Input: part model. Units: mm. Frame: model coordinates. Coordinates: 2 decimals unless noted, no trailing zeros. Order: outer loops, then holes, each group sorted by start corner. A loop starts at its lowest first (then second) coordinate and runs counter-clockwise, first axis right, second up. Notation, with made-up numbers: (71.25, 12) - (95.25, 12) arc R24 ccw to (95.25, 46) - close; hole circle Ø5 at (2.5, 55). An arc over 180 degrees is marked (long way). Answer as CSV lines item,"result". Start each with the question number.
Item 1: Draft query along X for faces 1 (the flat face through (26, 2, 6)), 2 (the cylindrical face through (47.79, -88.63, 2.96)), 3 (the cylindrical face through (-124.88, -5.5, 2.96)). Return one class per face: +X half, -X half, draft (parallel to the pull), parting line (faces both ways), or undercut.
Item 2: First-contact query: pin 1 (3.5 mm diameter, centred on x = -50, y = -86.6, fed in from -Z); pin 2 (1.5 mm diameter, centred on y = -67.5, z = 1, fed in from +X); pin 3 (1 mm diameter, centred on y = -99.5, z = 1.5, fed in from -X); pin 4 (1 mm diameter, centred on x = -27, z = 2, fed in from +Y). Flat tips, straight axial feed; report the tip coordinate or a pass-through.
Item 3: Section B-B (x = -76.95). Output: boundary loops of the cut face in (y, z).
Item 4: Material intervals for line 1 along Y through (x, z) = (-50.5, 0.75); line 2 along X through (y, z) = (41, 4.55); line 3 along Y through (x, z) = (-76.95, 1.75), sorted ascending.
Item 5: Section D-D (x = -50). Output: boundary loops of the cut face in (y, z).
Item 6: Section A-A (y = 0). Output: boundary loops of the cut face in (x, z), and give its area (3 significant figures).
Item 7: Section C-C (z = 1.4). State how many separate pieces and enclosed holes the cut face has, and give its area (3 significant figures).
Autodesk Fusion 360 part; units mm, degrees
sketch "Sketch1" plane through (0, 0, 0) normal (0, 0, 1) x (1, 0, 0)
  circle A0 centre (0, 0) radius 125
  line L0 (0, 0) -> (125, 0)
  line L1 (0, 0) -> (-62.5, -108.2532)
  line L2 (0, 0) -> (-62.5, 108.2532)
  line L3 (0, 0) -> (125, 0) construction
  line L4 (0, 0) -> (-25, 43.3013)
  line L5 (-25, 43.3013) -> (-50, 86.6025)
  line L6 (0, 0) -> (50, 0)
  line L7 (50, 0) -> (100, 0)
  line L8 (0, 0) -> (-25, -43.3013)
  line L9 (-25, -43.3013) -> (-50, -86.6025)
  circle A1 centre (-50, 86.6025) radius 3
  circle A2 centre (-25, 43.3013) radius 3
  circle A3 centre (50, 0) radius 3
  circle A4 centre (100, 0) radius 3
  circle A5 centre (-25, -43.3013) radius 3
  circle A6 centre (-50, -86.6025) radius 3
  line L10 (0, 0) -> (62.5, 108.2532)
  line L11 (0, 0) -> (125, 0) construction
  line L12 (0, 0) -> (62.5, -108.2532)
  line L13 (0, 0) -> (125, 0) construction
  line L14 (0, 0) -> (-125, 0)
  line L15 (0, 0) -> (-100, 0)
  circle A7 centre (-100, 0) radius 3
  line L16 (0, 0) -> (50, -86.6025)
  circle A8 centre (50, -86.6025) radius 3
  line L17 (0, 0) -> (50, 86.6025)
  circle A9 centre (50, 86.6025) radius 3
  circle A10 centre (0, 0) radius 3
  dimension "d1" = 250
  dimension "d2" = 60
  dimension "d3" = 120
  dimension "d4" = 50
  dimension "d5" = 50
  dimension "d6" = 50
  dimension "d7" = 50
  dimension "d8" = 50
  dimension "d9" = 50
  dimension "d10" = 6
  dimension "d11" = 6
  dimension "d12" = 6
  dimension "d13" = 6
  dimension "d14" = 6
  dimension "d15" = 6
  dimension "d16" = 60
  dimension "d17" = 60
  dimension "d18" = 100
  dimension "d19" = 6
  dimension "d20" = 100
  dimension "d21" = 6
  dimension "d22" = 100
  dimension "d23" = 6
  dimension "d24" = 6
extrude "Extrude1" add sketch "Sketch1" along normal blind 6 contours A0 L0 L6 L7 A3 A4 L10 L17 A9 A10 | A0 L0 L6 L7 A3 A4 L12 L16 A8 A10 | A0 L2 L4 L5 A1 A2 L10 L17 A9 A10 | A0 L1 L8 L9 A5 A6 L12 L16 A8 A10 | A0 L2 L4 L5 A1 A2 L14 L15 A7 A10 | A0 L1 L8 L9 A5 A6 L14 L15 A7 A10
sketch "Sketch2" plane through (0, 0, 6) normal (0, 0, 1) x (-1, 0, 0)
  circle A0 centre (0, 0) radius 3
  circle A1 centre (-50, -86.6025) radius 3
  circle A2 centre (25, -43.3013) radius 3
  circle A3 centre (100, 0) radius 3
  circle A4 centre (25, 43.3013) radius 3
  circle A5 centre (50, -86.6025) radius 3
  circle A6 centre (-100, 0) radius 3
  circle A7 centre (-50, 86.6025) radius 3
  circle A8 centre (-50, 0) radius 3
  circle A9 centre (50, 86.6025) radius 3
  circle A10 centre (0, 0) radius 125
  line L0 (125, 0) -> (115, 0)
  circle A11 centre (115, 0) radius 3
  circle A12 centre (105.0577, 46.7747) radius 3
  circle A13 centre (76.95, 85.4617) radius 3
  circle A14 centre (35.537, 109.3715) radius 3
  circle A15 centre (-12.0208, 114.37) radius 3
  circle A16 centre (-57.5, 99.5929) radius 3
  circle A17 centre (-93.037, 67.5953) radius 3
  circle A18 centre (-112.487, 23.9098) radius 3
  circle A19 centre (-112.487, -23.9098) radius 3
  circle A20 centre (-93.037, -67.5953) radius 3
  circle A21 centre (-57.5, -99.5929) radius 3
  circle A22 centre (-12.0208, -114.37) radius 3
  circle A23 centre (35.537, -109.3715) radius 3
  circle A24 centre (76.95, -85.4617) radius 3
  circle A25 centre (105.0577, -46.7747) radius 3
  dimension "d27" = 10
  dimension "d28" = 6
  dimension "d30" = 360
extrude "Extrude2" cut sketch "Sketch2" against normal blind 6 contours A11 | A12 | A13 | A14 | A15 | A16 | A17 | A18 | A19 | A20 | A21 | A22 | A23 | A24 | A25
sketch "Sketch3" plane through (0, 0, 6) normal (0, 0, 1) x (-1, 0, 0)
  circle A0 centre (35.537, 109.3715) radius 3
  circle A1 centre (-112.487, 23.9098) radius 3
  circle A2 centre (-12.0208, -114.37) radius 3
  circle A3 centre (115, 0) radius 3
  circle A4 centre (35.537, -109.3715) radius 3
  circle A5 centre (-112.487, -23.9098) radius 3
  circle A6 centre (-12.0208, 114.37) radius 3
  circle A7 centre (76.95, 85.4617) radius 3
  circle A8 centre (-93.037, 67.5953) radius 3
  circle A9 centre (-57.5, -99.5929) radius 3
  circle A10 centre (105.0577, -46.7747) radius 3
  circle A11 centre (76.95, -85.4617) radius 3
  circle A12 centre (-93.037, -67.5953) radius 3
  circle A13 centre (-57.5, 99.5929) radius 3
  circle A14 centre (105.0577, 46.7747) radius 3
  circle A15 centre (0, 0) radius 3
  circle A16 centre (-50, -86.6025) radius 3
  circle A17 centre (25, -43.3013) radius 3
  circle A18 centre (100, 0) radius 3
  circle A19 centre (25, 43.3013) radius 3
  circle A20 centre (50, -86.6025) radius 3
  circle A21 centre (-100, 0) radius 3
  circle A22 centre (-50, 86.6025) radius 3
  circle A23 centre (-50, 0) radius 3
  circle A24 centre (50, 86.6025) radius 3
  circle A25 centre (0, 0) radius 125
  line L0 (0, 0) -> (50, 0)
  line L1 (0, 0) -> (-50, -86.6025)
  line L2 (-50, 86.6025) -> (0, 0)
  circle A26 centre (-25, -43.3013) radius 3
  circle A27 centre (-25, 43.3013) radius 3
  circle A28 centre (50, 0) radius 3
  dimension "d33" = 50
  dimension "d34" = 6
  dimension "d35" = 6
  dimension "d36" = 6
extrude "Extrude3" cut sketch "Sketch3" against normal blind 6 contours L1 A26 | L1 A26 | L2 A27 | L2 A27 | A28
Determined:
1,face 1,"draft"
1,face 2,"undercut"
1,face 3,"parting line"
2,pin 1,"passes through"
2,pin 2,"stops at x = 105.69"
2,pin 3,"stops at x = -76.32"
2,pin 4,"stops at y = 122.16"
3,outline,"(-98.51, 0) - (-88.46, 0) - (-88.46, 6) - (-98.51, 6) - close; (-82.46, 0) - (82.46, 0) - (82.46, 6) - (-82.46, 6) - close; (88.46, 0) - (98.51, 0) - (98.51, 6) - (88.46, 6) - close"
4,line 1,"y = -114.34 to -89.56, -83.64 to -2.96, 2.96 to 83.64, 89.56 to 114.34"
4,line 2,"x = -118.08 to -26.92, -23.08 to 23.08, 26.92 to 118.08"
4,line 3,"y = -98.51 to -88.46, -82.46 to 82.46, 88.46 to 98.51"
5,outline,"(-114.56, 0) - (-89.6, 0) - (-89.6, 6) - (-114.56, 6) - close; (-83.6, 0) - (-3, 0) - (-3, 6) - (-83.6, 6) - close; (3, 0) - (83.6, 0) - (83.6, 6) - (3, 6) - close; (89.6, 0) - (114.56, 0) - (114.56, 6) - (89.6, 6) - close"
6,outline,"(-125, 0) - (-118, 0) - (-118, 6) - (-125, 6) - close; (-112, 0) - (-103, 0) - (-103, 6) - (-112, 6) - close; (-97, 0) - (-53, 0) - (-53, 6) - (-97, 6) - close; (-47, 0) - (-3, 0) - (-3, 6) - (-47, 6) - close; (3, 0) - (47, 0) - (47, 6) - (3, 6) - close; (53, 0) - (97, 0) - (97, 6) - (53, 6) - close; (103, 0) - (125, 0) - (125, 6) - (103, 6) - close"
6,area,"1,280 mm^2"
7,separate pieces,"1"
7,enclosed holes,"28"
7,area,"48,300 mm^2"
